Read the model definition and answer for the solid it produces. Units are mm, in the model's axes. A direction names the side the tool comes from. Coordinates: 2 decimals unless noted, no trailing zeros. Order: outer loops, then holes, each group sorted by start corner. A loop starts at its lowest first (then second) coordinate and runs counter-clockwise, first axis right, second up. Notation, with made-up numbers: (-7.75, 18.25) - (51.25, 18.25) arc R20 cw to (51.25, 41.25) - close; hole circle Ø1 at (27, 44). An arc over 180 degrees is marked (long way). Write item = value, one per line.
from build123d import *

# Parameters (mm, degrees)
BOSS_EXTRUDE1_DEPTH = 3.175
SWEEP1_PROFILE_R    = 1.5875
FILLET1_R           = 3.81
SKETCH14_W          = 49.53
SKETCH14_H          = 3.81
BOSS_EXTRUDE4_DEPTH = 3.175
FILLET2_R           = 2.54
FILLET4_R           = 2.54
SKETCH15_W          = 46.99
SKETCH15_H          = 74.422
SKETCH15_W_2        = 40.64
SKETCH15_H_2        = 68.072
BOSS_EXTRUDE6_DEPTH = 3.175


# Some blends are built 0.0001 mm under size
with BuildPart() as part:
    # Sketch1 → Boss-Extrude1 (new body)
    with BuildSketch(Plane.XY):
        Polygon((-24.765, -37.211), (24.765, -37.211), (24.765, -18.570359608), (24.765, 0.678999912), (24.765, 37.211), (-24.765, 37.211), (-24.765, 0.678999912), (-24.765, -18.570359608), align=None)
    extrude(amount=BOSS_EXTRUDE1_DEPTH)

    # Sweep1: sweep along a path in Sketch7
    with BuildLine(Plane(origin=(0, -5.770679848, 0), x_dir=(1, 0, 0), z_dir=(0, 1, 0))) as sweep1_path:
        Line((-12.7, -3.175), (-12.7, -6.985))
        ThreePointArc((-12.7, -6.985), (0, -19.685), (12.7, -6.985))
        Line((12.7, -6.985), (12.7, -3.175))
    # Sweep1 profile (on start of the path) → Sweep1 (sweep)
    with BuildSketch(Plane(origin=(-12.7, -5.770679848, 3.175), x_dir=(1, 0, 0), z_dir=(0, 0, 1))):
        Circle(SWEEP1_PROFILE_R)
    sweep(path=sweep1_path.line)

    # Fillet1
    fillet1_edges = [part.edges().sort_by_distance(p)[0] for p in [
        (14.2875, -5.770679848, 3.175),
        (-14.2875, -5.770679848, 3.175),
    ]]
    fillet(fillet1_edges, radius=FILLET1_R - 0.0001)  # a hair under: the kernel refuses the full size

    # Sketch14 → Boss-Extrude4 (add)
    with BuildSketch(Plane.XY.offset(3.175)):
        with Locations((0, -39.116)):
            Rectangle(SKETCH14_W, SKETCH14_H)
        with Locations((0, 39.116)):
            Rectangle(SKETCH14_W, SKETCH14_H)
    extrude(amount=-BOSS_EXTRUDE4_DEPTH)

    # Fillet2
    fillet2_edges = [part.edges().sort_by_distance(p)[0] for p in [
        (-24.765, 0, 3.175),
        (0, -41.021, 3.175),
        (24.765, 0, 3.175),
        (0, 41.021, 3.175),
    ]]
    fillet(fillet2_edges, radius=FILLET2_R)

    # Fillet4
    # the kernel refuses this fillet: 2.54 mm, written as the material it takes off along each edge
    with BuildSketch(Plane(origin=(-22.225, -38.481, 0.635), x_dir=(0, -1, 0), z_dir=(-1, 0, 0))) as fillet4_piece_1_section:
        Polygon((0, 0), (FILLET4_R, 0), (FILLET4_R, FILLET4_R), (0, FILLET4_R), align=None)
    fillet4_piece_1 = extrude(amount=FILLET4_R, mode=Mode.PRIVATE)
    fillet4_piece_1 = fillet4_piece_1 - Plane(origin=(-22.225, -38.481, 0.635), x_dir=(0, 0.7071067811865475, -0.7071067811865475), z_dir=(-1, 0, 0)) * Sphere(FILLET4_R, mode=Mode.PRIVATE)
    add(fillet4_piece_1, mode=Mode.SUBTRACT)
    with BuildSketch(Plane(origin=(-22.225, 38.481, 0.635), x_dir=(0, 1, 0), z_dir=(-1, 0, 0))) as fillet4_piece_2_section:
        Polygon((0, 0), (FILLET4_R, 0), (FILLET4_R, -FILLET4_R), (0, -FILLET4_R), align=None)
    fillet4_piece_2 = extrude(amount=FILLET4_R, mode=Mode.PRIVATE)
    fillet4_piece_2 = fillet4_piece_2 - Plane(origin=(-22.225, 38.481, 0.635), x_dir=(0, -0.7071067811865475, -0.7071067811865475), z_dir=(-1, 0, 0)) * Sphere(FILLET4_R, mode=Mode.PRIVATE)
    add(fillet4_piece_2, mode=Mode.SUBTRACT)
    with BuildSketch(Plane(origin=(22.225, -38.481, 0.635), x_dir=(1, 0, 0), z_dir=(0, -1, 0))) as fillet4_piece_3_section:
        Polygon((0, 0), (FILLET4_R, 0), (FILLET4_R, FILLET4_R), (0, FILLET4_R), align=None)
    fillet4_piece_3 = extrude(amount=FILLET4_R, mode=Mode.PRIVATE)
    fillet4_piece_3 = fillet4_piece_3 - Plane(origin=(22.225, -38.481, 0.635), x_dir=(-0.7071067811865475, 1.0781380386361295e-15, -0.7071067811865475), z_dir=(0, -1, 0)) * Sphere(FILLET4_R, mode=Mode.PRIVATE)
    add(fillet4_piece_3, mode=Mode.SUBTRACT)
    with BuildSketch(Plane(origin=(22.225, 38.481, 0.635), x_dir=(1, 0, 0), z_dir=(0, 1, 0))) as fillet4_piece_4_section:
        Polygon((0, 0), (FILLET4_R, 0), (FILLET4_R, -FILLET4_R), (0, -FILLET4_R), align=None)
    fillet4_piece_4 = extrude(amount=FILLET4_R, mode=Mode.PRIVATE)
    fillet4_piece_4 = fillet4_piece_4 - Plane(origin=(22.225, 38.481, 0.635), x_dir=(-0.7071067811865475, 1.0781380386361295e-15, -0.7071067811865475), z_dir=(0, 1, 0)) * Sphere(FILLET4_R, mode=Mode.PRIVATE)
    add(fillet4_piece_4, mode=Mode.SUBTRACT)
    with BuildSketch(Plane(origin=(24.765, -41.021, 0.635), x_dir=(-1, 0, 0), z_dir=(0, 0, -1)), Plane(origin=(-24.765, -41.021, 0.635), x_dir=(0, 1, 0), z_dir=(0, 0, -1))) as fillet4_piece_5:
        with BuildLine():
            CenterArc((FILLET4_R, FILLET4_R), FILLET4_R, 180, 90)
            Line((0, FILLET4_R), (0, 0))
            Line((0, 0), (FILLET4_R, 0))
        make_face()
    extrude(amount=6.985, mode=Mode.SUBTRACT)
    with BuildSketch(Plane(origin=(24.765, 41.021, 0.635), x_dir=(-1, 0, 0), z_dir=(0, 0, -1)), Plane(origin=(-24.765, 41.021, 0.635), x_dir=(0, -1, 0), z_dir=(0, 0, -1))) as fillet4_piece_6:
        with BuildLine():
            CenterArc((FILLET4_R, -FILLET4_R), FILLET4_R, 90, 90)
            Line((0, -FILLET4_R), (0, 0))
            Line((0, 0), (FILLET4_R, 0))
        make_face()
    extrude(amount=6.985, mode=Mode.SUBTRACT)

    # Sketch15 → Boss-Extrude6 (add)
    with BuildSketch(Plane(origin=(0, 0, 0), x_dir=(-1, 0, 0), z_dir=(0, 0, -1))):
        Rectangle(SKETCH15_W, SKETCH15_H)
        Rectangle(SKETCH15_W_2, SKETCH15_H_2, mode=Mode.SUBTRACT)
    extrude(amount=BOSS_EXTRUDE6_DEPTH)


solid = part.part
1) Determine the mould class of faces 1 (the face through (-24, -40.3, 0.3)), 2 (the face through (0, 0, 0)), 3 (the face through (-24, 40.3, 0.3)), 4 (the face through (-24, 0, 0)) for opening direction Y: pulls with the +Y half, pulls with the -Y half, needs draft (parallel to the pull), parting line crosses it, or undercut.
Returned:
face_1 = pulls with the -Y half
face_2 = undercut
face_3 = pulls with the +Y half
face_4 = needs draft
2) For faces 5 (the face through (-23.495, -1, -2)), 6 (the face through (0, -37.211, -2)), 7 (the face through (-20.32, 0, -2)), 8 (the face through (23.495, -1, -2)), determine the directions among +Z, -Z, +X, -X, +Y, -Y from which every point of the face is accessible in a straight line to the end or side of a thin tool.
Returned:
face_5 = -Z, -X, +Y, -Y
face_6 = -Z, +X, -X, -Y
face_7 = -Z
face_8 = -Z, +X, +Y, -Y
3) Straight lines are drawn through the part: line 1 along Y through (x, z) = (13, -1.25); line 2 along Z through (x, y) = (-19.5, 10) (3 decimals); line 3 along Z through (x, y) = (-3, 37) (3 decimals). For each, find the intervals that lie inside material, in ascending order. Write a range as from..to.
Returned:
line_1 = -37.21..-34.04, 34.04..37.21
line_2 = 0..3.175
line_3 = -3.175..3.175
4) Flat-ended cylindrical pins translate along their axes: pin 1 Ø22 at (x, y) = (-10.5, 8) entering from +Z; pin 2 Ø2.5 at (y, z) = (9.5, -2) entering from -X (3 decimals); pin 3 Ø2 at (y, z) = (25, 2) entering from +X; pin 4 Ø8 at (y, z) = (25, 11) entering from -X. Find the tip coordinate at first contact, or state that the pin passes through.
Returned:
pin_1 = 4.07
pin_2 = -23.495
pin_3 = 24.74
pin_4 = through
5) The part is cut by section B-B (z = 4). Determine the outline of the cut face in (x, y), and give its area (3 significant figures).
Returned:
outline = circle Ø6.06 at (-12.7, -5.77); circle Ø6.06 at (12.7, -5.77)
area = 57.7 mm^2
6) The part is cut by section A-A (y = 15.5). Determine the outline of the cut face in (x, z) (3 decimals).
Returned:
outline = (-24.765, 0) - (-23.495, 0) - (-23.495, -3.175) - (-20.32, -3.175) - (-20.32, 0) - (20.32, 0) - (20.32, -3.175) - (23.495, -3.175) - (23.495, 0) - (24.765, 0) - (24.765, 0.635) arc R2.54 ccw to (22.225, 3.175) - (-22.225, 3.175) arc R2.54 ccw to (-24.765, 0.635) - close
